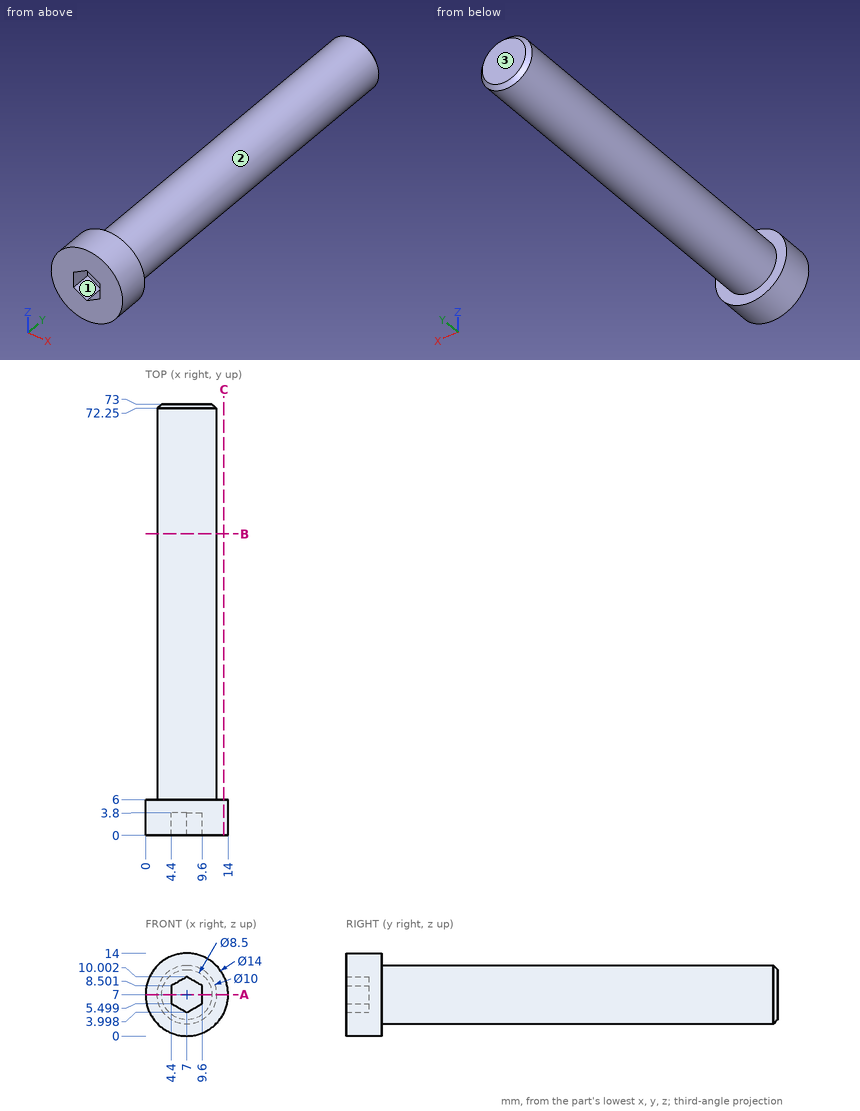
Job drawing, mm, ordinate dimensions from the low corner. One solid piece. Coordinates: 2 decimals unless noted, no trailing zeros. Order: outer loops, then holes, each group sorted by start corner. A loop starts at its lowest first (then second) coordinate and runs counter-clockwise, first axis right, second up. Notation, with made-up numbers: (-21.5, -6) -> (29.5, -6) arc R19 cw to (29.5, 30) -> close; hole circle Ø10 at (29.5, 39.5). An arc over 180 degrees is marked (long way). Answer in a Markdown table with one row per item. Add a question column.
Q1. Band-saw the part on B-B, the plane y = 51. List the corners of the cut face in (x, z).
Q2. Drop flat-ended pins along their axis: pin 1 (5 mm diameter, centred on x = 3.5, y = 55.5, fed in from -Z); pin 2 (3 mm diameter, centred on y = 34.5, z = 10, fed in from +X); pin 3 (6 mm diameter, centred on x = 10.5, y = 21, fed in from +Z) (3 decimals). Give the stop position or say it passes through.
Q3. Band-saw the part on A-A, the plane z = 7. List the corners of the cut face in (x, y), then the cut area to 3 significant figures.
Q4. Band-saw the part on C-C, the plane x = 13.25. List the corners of the cut face in (y, z).
Q5. Mould opens along Z. For the marked faces 1, 2 and 3 say: +Z half, -Z half, draft (parallel to the pull), parting line (faces both ways), or undercut.
Q6. Wall check: line 1 along Y through (x, z) = (6.5, 5.25); line 2 along X through (y, z) = (21.5, 7.25); line 3 along Y through (x, z) = (0.75, 4.25). Give the ranges that are in metal, low to high. Write a range as [from, to].
Answers follow:
| question | item | result |
|---|---|---|
| 1 | outline | circle Ø10 at (7, 7) |
| 2 | pin 1 | z = 2.1 |
| 2 | pin 2 | x = 11.77 |
| 2 | pin 3 | z = 11.975 |
| 3 | outline | (0, 0) -> (4.4, 0) -> (4.4, 3.8) -> (9.6, 3.8) -> (9.6, 0) -> (14, 0) -> (14, 6) -> (12, 6) -> (12, 72.25) -> (11.25, 73) -> (2.75, 73) -> (2, 72.25) -> (2, 6) -> (0, 6) -> close |
| 3 | area | 734 mm^2 |
| 4 | outline | (0, 3.85) -> (6, 3.85) -> (6, 10.15) -> (0, 10.15) -> close |
| 5 | face 1 | undercut |
| 5 | face 2 | parting line |
| 5 | face 3 | draft |
| 6 | line 1 | [3.8, 73] |
| 6 | line 2 | [2.01, 11.99] |
| 6 | line 3 | [0, 6] |
